Autodesk Inventor part; units mm, degrees
ref_plane "YZ Plane" through (0, 0, 0) normal (1, 0, 0) x (0, 1, 0)
ref_plane "XZ Plane" through (0, 0, 0) normal (0, 1, 0) x (-1, 0, 0)
ref_plane "XY Plane" through (0, 0, 0) normal (0, 0, 1) x (1, 0, 0)
sketch "Sketch1" plane through (0, 0, 0) normal (0, 1, 0) x (-1, 0, 0)
  line L0 (0, 0) -> (101.6, 0)
  line L1 (101.6, 0) -> (101.6, 25.4)
  line L2 (101.6, 25.4) -> (0, 25.4)
  line L3 (0, 25.4) -> (0, 0)
  dimension "d0" = 101.6
  dimension "d1" = 25.4
extrude "Extrusion1" add sketch "Sketch1" along normal blind 50.8
sketch "Sketch2" plane through (-101.6, 0, 25.4) normal (0, 0, 1) x (1, 0, 0)
  circle A0 centre (50.8, 25.4) radius 4.7625
  line L0 (101.6, 50.8) -> (0, 50.8)
  line L1 (101.6, 0) -> (101.6, 50.8)
  dimension "d4" = 9.525
  dimension "d5" = 25.4
  dimension "d6" = 50.8
extrude "Extrusion2" cut sketch "Sketch2" against normal blind 111.125
sketch "Sketch3" plane through (0, 0, 25.4) normal (1, 0, 0) x (0, 0, -1)
  line L0 (3.175, 3.175) -> (22.225, 3.175)
  line L1 (22.225, 3.175) -> (22.225, 47.625)
  line L2 (22.225, 47.625) -> (3.175, 47.625)
  line L3 (3.175, 47.625) -> (3.175, 3.175)
  line L4 (0, 0) -> (0, 50.8)
  line L5 (0, 0) -> (25.4, 0)
  line L6 (25.4, 0) -> (25.4, 50.8)
  line L7 (25.4, 50.8) -> (0, 50.8)
  dimension "d9" = 3.175
  dimension "d10" = 3.175
  dimension "d11" = 3.175
  dimension "d12" = 3.175
extrude "Extrusion3" cut sketch "Sketch3" against normal blind 111.125 contours L3 L2 L1 L0
sketch "Sketch4" plane through (0, 50.8, 0) normal (0, 1, 0) x (1, 0, 0)
  circle A0 centre (-12.7, -12.827) radius 2.54
  circle A1 centre (-88.9, -12.827) radius 2.54
  line L0 (0, 0) -> (-101.6, 0)
  line L1 (-101.6, 0) -> (-101.6, -25.4)
  line L2 (0, -25.4) -> (0, 0)
  dimension "d15" = 5.08
  dimension "d16" = 12.827
  dimension "d17" = 12.7
  dimension "d18" = 5.08
  dimension "d19" = 12.827
  dimension "d20" = 12.7
  dimension "d21" = 76.2
extrude "Extrusion4" cut sketch "Sketch4" against normal blind 111.125
properties part number "15102898-16-P-0306"
Here's how the part is built. I have some questions about the finished solid (model axes, mm). A direction names the side the tool comes from. Round coordinates to 2 decimals unless told otherwise and drop trailing zeros. Loops run counter-clockwise (first coordinate to the right, second up) from the corner with the lowest first, then second, coordinate; pieces in that order, holes last. Notation, with made-up numbers: (88, 3) -> (118, 3) arc R21 cw to (118, 11) -> close; hole circle Ø9 at (31.25, 69). An arc over 180 degrees is marked (long way). Answer as CSV lines item,"result". Start each with the question number.
1. Imagine slicing it at A-A on x = -50.8. Write out the boundary of the cut face in (y, z) (1 decimal).
2. If we mould it in two halves opening along X, with no side actions, what happens to faces 3 (the face through (-50, 31, 22.225)), 4 (the face through (-55.558, 25.609, 1.61)), 5 (the face through (-101.6, 27, 2))? For each: pulls with the +X half, pulls with the -X half, needs draft (parallel to the pull), parting line crosses it, or undercut.
3. For faces 1 (the face through (-50, 3.175, 13)), 2 (the face through (-50, 0, 13)), which set-ups out of +Z, -Z, +X, -X, +Y, -Y let a thin tool reach every point of the face, with its end or its side?
4. Imagine slicing it at D-D on x = -95. Write out the boundary of the cut face in (y, z) (3 decimals), plus the area to 3 significant figures.
5. I need wall thicknesses on probe 1 along Y at (x, z) = (-80, 12.75) (3 decimals); probe 2 along Z at (x, y) = (-34.5, 44.5) (3 decimals); probe 3 along Z at (x, y) = (-12, 2). Which ranges of each line are inside material? Lowest first, please. Write a range as from..to.
6. Imagine slicing it at B-B on z = 7.5. Write out the boundary of the cut face in (x, y) (3 decimals), plus the area to 3 significant figures.
7. Imagine slicing it at C-C on y = 25.4. Write out the boundary of the cut face in (x, z) (1 decimal), plus the area to 3 significant figures.
8. I'm going to push a flat-ended pin straight in: P1, Ø10, axis at y = 20, z = 19, coming from the +X side. Where does the tip first touch, or does it pass through?
Solution:
1,outline,"(0, 0) -> (20.6, 0) -> (20.6, 3.2) -> (3.2, 3.2) -> (3.2, 22.2) -> (20.6, 22.2) -> (20.6, 25.4) -> (0, 25.4) -> close; (30.2, 0) -> (50.8, 0) -> (50.8, 25.4) -> (30.2, 25.4) -> (30.2, 22.2) -> (47.6, 22.2) -> (47.6, 3.2) -> (30.2, 3.2) -> close"
2,face 3,"needs draft"
2,face 4,"undercut"
2,face 5,"pulls with the -X half"
3,face 1,"+X, -X"
3,face 2,"+Z, -Z, +X, -X, -Y"
4,outline,"(0, 0) -> (50.8, 0) -> (50.8, 25.4) -> (0, 25.4) -> close; hole (3.175, 3.175) -> (47.625, 3.175) -> (47.625, 22.225) -> (3.175, 22.225) -> close"
4,area,"444 mm²"
5,probe 1,"0..3.175, 47.625..50.8"
5,probe 2,"0..3.175, 22.225..25.4"
5,probe 3,"0..10.39, 15.27..25.4"
6,outline,"(-101.6, 0) -> (0, 0) -> (0, 3.175) -> (-101.6, 3.175) -> close; (-101.6, 47.625) -> (0, 47.625) -> (0, 50.8) -> (-101.6, 50.8) -> close"
6,area,"645 mm²"
7,outline,"(-101.6, 0) -> (-55.6, 0) -> (-55.6, 3.2) -> (-101.6, 3.2) -> close; (-101.6, 22.2) -> (-55.6, 22.2) -> (-55.6, 25.4) -> (-101.6, 25.4) -> close; (-46, 0) -> (0, 0) -> (0, 3.2) -> (-46, 3.2) -> close; (-46, 22.2) -> (0, 22.2) -> (0, 25.4) -> (-46, 25.4) -> close"
7,area,"585 mm²"
8,P1,"x = 0"
